For this review, use the dimensioned drawing (mm, ordinates from the lowest corner) and the shaded views. Coordinates: 2 decimals unless noted, no trailing zeros. Write each loop counter-clockwise with the first axis right and the second up, starting at its lowest first coordinate (ties: lowest second). Pieces come first, ordered by that corner, then holes. Notation, with made-up numbers: (32, 25) -> (75, 25) arc R25 ccw to (75, 49) -> close; hole circle Ø5 at (40.5, 14.25). An arc over 180 degrees is marked (long way). Return JSON: item names as keys, results as strings. Group by question number.
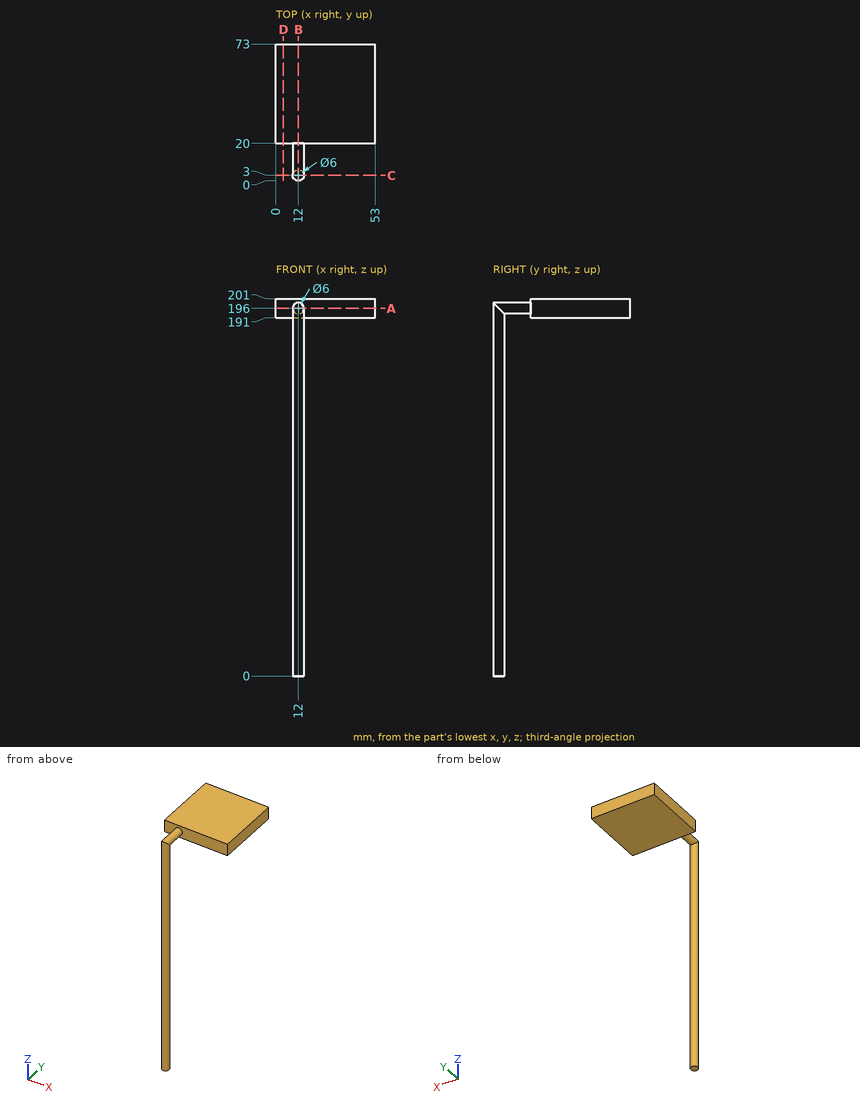
Q1. For P1, Ø11, axis at x = 27.5, z = 196, coming from the -Y side; P2, Ø4, axis at x = 36.5, y = 37.5, coming from the -Z side, all flat-tipped, find the tip position at first contact; note any pin that passes through.
Q2. We need section A-A on z = 196. Write out the cut boundary in (x, y).
Q3. We need section D-D on x = 4. Write out the cut boundary in (y, z).
Q4. Wall thickness on L1, parallel to Z at x = 21.5, y = 33; L2, parallel to Z at x = 13, y = 14; L3, parallel to Y at x = 14, z = 69.5: over which ranges is each line inside the solid? List them lowest first.
Q5. We need section B-B on x = 12. Write out the cut boundary in (y, z), plus the area to 3 significant figures.
Q6. We need section C-C on y = 3. Write out the cut boundary in (x, z), plus the area to 3 significant figures.
Findings below:
{
 "1": {"P1": "stops at y = 20", "P2": "stops at z = 191"},
 "2": {"outline": "(0, 20) -> (9, 20) -> (9, 3) arc R3 ccw to (15, 3) -> (15, 20) -> (53, 20) -> (53, 73) -> (0, 73) -> close"},
 "3": {"outline": "(20, 191) -> (73, 191) -> (73, 201) -> (20, 201) -> close"},
 "4": {"L1": "z = 191 to 201", "L2": "z = 193.17 to 198.83", "L3": "y = 0.76 to 5.24"},
 "5": {"outline": "(0, 0) -> (6, 0) -> (6, 193) -> (20, 193) -> (20, 191) -> (73, 191) -> (73, 201) -> (20, 201) -> (20, 199) -> (0, 199) -> close", "area": "1,810 mm^2"},
 "6": {"outline": "(9, 0) -> (15, 0) -> (15, 196) arc R3 ccw to (9, 196) -> close", "area": "1,190 mm^2"}
}
